For this review, take the finished solid that the model builds, in its own axes (mm). A direction names the side the tool comes from. Give positions to 0.01 mm unless a question says otherwise; leave off trailing zeros. Loops run counter-clockwise (first coordinate to the right, second up) from the corner with the lowest first, then second, coordinate; pieces in that order, holes last.
Autodesk Inventor part; units mm, degrees
ref_plane "YZ Plane" through (0, 0, 0) normal (1, 0, 0) x (0, 1, 0)
ref_plane "XZ Plane" through (0, 0, 0) normal (0, 1, 0) x (-1, 0, 0)
ref_plane "XY Plane" through (0, 0, 0) normal (0, 0, 1) x (1, 0, 0)
sketch "Sketch1" plane through (0, 0, 0) normal (1, 0, 0) x (0, 1, 0)
  line L0 (0, 0) -> (40, 0) construction
  line L1 (40, 0) -> (40, 66.5) construction
  line L2 (40, 66.5) -> (0, 66.5) construction
  line L3 (0, 66.5) -> (0, 0) construction
  line L4 (0, 66.5) -> (40, 66.5) construction
  line L5 (40, 66.5) -> (40, 86.5) construction
  line L6 (40, 86.5) -> (0, 86.5)
  line L7 (0, 86.5) -> (0, 66.5) construction
  line L8 (0, 0) -> (40, 0) construction
  line L9 (40, 0) -> (40, -20) construction
  line L10 (40, -20) -> (0, -20) construction
  line L11 (0, -20) -> (0, 0) construction
  line L12 (48.2, 61.45) -> (-8.2, 61.45) construction
  line L13 (-8.2, 61.45) -> (-8.2, 5.05) construction
  line L14 (-8.2, 5.05) -> (48.2, 5.05) construction
  line L15 (48.2, 5.05) -> (48.2, 61.45) construction
  line L16 (48.2, 33.25) -> (-8.2, 33.25) construction
  line L17 (40, 33.25) -> (0, 33.25) construction
  line L18 (43.57, 56.82) -> (-3.57, 56.82) construction
  line L19 (-3.57, 56.82) -> (-3.57, 9.68) construction
  line L20 (-3.57, 9.68) -> (43.57, 9.68) construction
  line L21 (43.57, 9.68) -> (43.57, 56.82) construction
  line L22 (43.57, 56.82) -> (48.2, 56.82) construction
  line L23 (43.57, 56.82) -> (43.57, 61.45) construction
  line L24 (-3.57, 9.68) -> (-8.2, 9.68) construction
  line L25 (-3.57, 9.68) -> (-3.57, 5.05) construction
  line L26 (40, -10) -> (0, -10) construction
  line L27 (40, 76.5) -> (0, 76.5) construction
  circle A0 centre (30, 76.5) radius 2.1
  circle A1 centre (10, 76.5) radius 2.1
  circle A2 centre (30, -10) radius 2.1
  circle A3 centre (10, -10) radius 2.1
  circle A4 centre (43.57, 56.82) radius 2.6
  circle A5 centre (43.57, 9.68) radius 2.6
  circle A6 centre (-3.57, 9.68) radius 2.6
  circle A7 centre (-3.57, 56.82) radius 2.6
  circle A8 centre (20, 33.25) radius 19.15
  circle A9 centre (-25, 18.25) radius 11.08 construction
  circle A10 centre (-25, 18.25) radius 13 construction
  circle A11 centre (-25, 18.25) radius 2.5
  line L28 (-60, 153.25) -> (-60, -86.75) construction
  circle A12 centre (-60, -86.75) radius 2.6
  circle A13 centre (-60, 153.25) radius 2.6
  line L29 (-120.2, 153.25) -> (-120.2, -86.75) construction
  circle A14 centre (-120.2, -86.75) radius 2.6
  circle A15 centre (-120.2, 153.25) radius 2.6
  circle A16 centre (-60, -86.75) radius 12 construction
  circle A17 centre (-120.2, -86.75) radius 12 construction
  circle A18 centre (-120.2, 153.25) radius 12 construction
  circle A19 centre (-60, 153.25) radius 12 construction
  line L30 (-110, 482.7599) -> (-70, 482.7599) construction
  line L31 (-70, -517.2401) -> (-110, -517.2401) construction
  circle A20 centre (-25, 48.25) radius 2.5
  circle A21 centre (-25, 48.25) radius 11.08 construction
  circle A22 centre (-25, 48.25) radius 13 construction
  circle A23 centre (20, 33.25) radius 11.08 construction
  circle A24 centre (20, 33.25) radius 13 construction
  line L32 (-23.1873, 29.1807) -> (18.1873, 22.3193) construction
  line L33 (18.1873, 44.1807) -> (-23.1873, 37.3193) construction
  line L34 (-120.8333, -99.25) -> (-47.8333, -99.25)
  line L35 (-47.8333, 165.75) -> (-120.8333, 165.75)
  line L36 (-132.8333, 153.75) -> (-132.8333, -87.25)
  line L37 (-60, 153.25) -> (-120.2, 153.25) construction
  line L38 (-120.2, -86.75) -> (-60, -86.75) construction
  line L39 (-60, 153.25) -> (-60, 165.75) construction
  line L40 (-120.2, -86.75) -> (-120.2, -99.25) construction
  line L41 (48.3276, -20) -> (48.3276, 86.5)
  line L42 (17.6122, 86.5) -> (40, 86.5) construction
  arc A25 (-120.8333, 165.75) -> (-132.8333, 153.75) centre (-120.8333, 153.75) ccw
  arc A26 (-132.8333, -87.25) -> (-120.8333, -99.25) centre (-120.8333, -87.25) ccw
  line L43 (48.3276, -20) -> (-47.8333, -99.25)
  line L44 (-47.8333, 165.75) -> (-47.8333, -99.25) construction
  line L45 (-120.2, -86.75) -> (-132.8333, -86.75) construction
  line L46 (-60, 153.25) -> (-47.8333, 153.25) construction
  line L47 (-36.08, 48.25) -> (-36.08, 286.613) construction
  line L48 (-47.8333, 145.75) -> (-47.8333, 86.5)
  line L49 (-47.8333, 86.5) -> (16.8804, 86.5)
  line L50 (-47.8333, -73.3332) -> (16.8804, -20)
  line L51 (-47.8333, -73.3332) -> (-47.8333, -20)
  line L52 (-47.8333, -20) -> (16.8804, -20)
  line L53 (48.3276, 86.5) -> (48.3276, 165.75)
  line L54 (48.3276, 165.75) -> (-47.8333, 165.75)
  line L55 (-47.8333, 145.75) -> (28.3276, 145.75)
  line L56 (28.3276, 145.75) -> (28.3276, 86.5)
  line L57 (-47.8333, 145.75) -> (28.3276, 86.5) construction
  line L58 (-39.6904, 145.75) -> (28.3276, 92.8349)
  line L59 (-47.8333, 139.4151) -> (20.1847, 86.5)
  point P0 (-132.8333, -99.25)
  point P1 (-132.8333, 165.75)
  point P2 (-47.8333, 139.8332)
  point P3 (0, 86.5)
  dimension "d25" = 22.16
  dimension "d0" = 40
  dimension "d1" = 66.5
  dimension "d2" = 40
  dimension "d3" = 20
  dimension "d4" = 40
  dimension "d5" = 20
  dimension "d6" = 56.4
  dimension "d7" = 56.4
  dimension "d8" = 0
  dimension "d9" = 8.2
  dimension "d10" = 47.14
  dimension "d11" = 47.14
  dimension "d12" = 4.2
  dimension "d13" = 20
  dimension "d14" = 10
  dimension "d15" = 10
  dimension "d16" = 20
  dimension "d17" = 4.2
  dimension "d18" = 4.2
  dimension "d19" = 4.2
  dimension "d20" = 5.2
  dimension "d21" = 5.2
  dimension "d22" = 5.2
  dimension "d23" = 5.2
  dimension "d24" = 38.3
  dimension "d26" = 26
  dimension "d27" = 5
  dimension "d28" = 240
  dimension "d30" = 60
  dimension "d31" = 5.2
  dimension "d32" = 5.2
  dimension "d33" = 5.2
  dimension "d34" = 5.2
  dimension "d35" = 60.2
  dimension "d36" = 24
  dimension "d37" = 24
  dimension "d38" = 24
  dimension "d39" = 24
  dimension "d40" = 40
  dimension "d41" = 1000
  dimension "d44" = 45
  dimension "d45" = 5
  dimension "d46" = 22.16
  dimension "d47" = 26
  dimension "d48" = 45
  dimension "d49" = 22.16
  dimension "d50" = 26
  dimension "d51" = 15
  dimension "d52" = 15
  dimension "d53" = 265
  dimension "d54" = 85
  dimension "d55" = 106.5
  dimension "d60" = 12
  dimension "d84" = 72.8333
  dimension "d87" = 28.3276
  dimension "d90" = 53.25
  dimension "d91" = 85
  dimension "d92" = 132.5
  dimension "d93" = 60.2
  dimension "d99" = 20
  dimension "d100" = 20
  dimension "d102" = 5
  dimension "d103" = 5
extrude "Extrusion1" add sketch "Sketch1" along normal blind 3.175 contours L6 L59 L48 L55 L58 L56 | A26 L36 A25 L35 L54 L53 L41 L43 L34
sketch "Sketch4" plane through (3.175, 0, 0) normal (1, 0, 0) x (0, 0, -1)
  line L0 (20, 16.8804) -> (73.3332, -47.8333)
  line L1 (20, 16.8804) -> (73.3332, -47.8333)
  line L2 (39.0796, -6.2705) -> (54.5136, 6.4492) construction
  line L3 (99.25, -47.8333) -> (20, 48.3276)
  circle A0 centre (37.2568, 11.6648) radius 2.6
  circle A1 centre (56.3364, -11.4861) radius 2.6
  line L4 (37.2568, 11.6648) -> (46.7966, 0.0893) construction
  line L5 (56.3364, -11.4861) -> (46.7966, 0.0893) construction
  line L6 (-145.75, 28.3276) -> (-92.8349, 28.3276)
  line L7 (-119.2924, 28.3276) -> (-119.2924, 48.3276) construction
  line L8 (20, 48.3276) -> (-165.75, 48.3276) construction
  circle A2 centre (-104.2924, 38.3276) radius 2.6
  circle A3 centre (-134.2924, 38.3276) radius 2.6
  line L9 (-104.2924, 38.3276) -> (-119.2924, 38.3276) construction
  line L10 (-134.2924, 38.3276) -> (-119.2924, 38.3276) construction
  point P0 (0, 0)
  dimension "d107" = 5.2
  dimension "d108" = 5.2
  dimension "d109" = 15
  dimension "d110" = 15
  dimension "d111" = 30
  dimension "d112" = 5.2
  dimension "d113" = 5.2
  dimension "d114" = 15
  dimension "d115" = 15
extrude "Extrusion4" cut sketch "Sketch4" against normal through all
fillet "Fillet2" radius 3.175 7 edges at (1.5875, -47.8333, 139.4151) (1.5875, -47.8333, 86.5) (1.5875, -47.8333, -20) (1.5875, -47.8333, -73.3332) (1.5875, 16.8804, -20) (1.5875, 48.3276, -20) (1.5875, -47.8333, -99.25)
fillet "Fillet3" radius 3.175 4 edges at (1.5875, 28.3276, 145.75) (1.5875, 28.3276, 92.8349) (1.5875, 20.1847, 86.5) (1.5875, -39.6904, 145.75)
chamfer "Chamfer1" distance 10 angle 45 1 edges at (1.5875, 48.3276, 165.75)
equation "\"d11\" = d10"
equation "\"d17\" = d12"
equation "\"d18\" = d12"
equation "\"d19\" = d12"
equation "\"d21\" = d20"
equation "\"d22\" = d20"
equation "\"d23\" = d20"
equation "\"d32\" = d31"
equation "\"d33\" = d31"
equation "\"d34\" = d31"
equation "\"d37\" = d36"
equation "\"d38\" = d36"
equation "\"d39\" = d36"
equation "\"d45\" = d27"
equation "\"d46\" = d25"
equation "\"d47\" = d26"
properties part number "X Axis V Wheel and Motor Frame Machined"
Item 1: Take a section at B-B on z = 123.5. Give the boundary of the cut face in (x, y) (3 decimals).
Answer:
outline: (0, -132.833) - (3.175, -132.833) - (3.175, -47.833) - (0, -47.833) - close; (0, -27.376) - (3.175, -27.376) - (3.175, -11.09) - (0, -11.09) - close; (0, 28.328) - (3.175, 28.328) - (3.175, 48.328) - (0, 48.328) - close
Item 2: Tool access review of faces 1 (the flat face through (1.565, -15.302, 114.107)), 2 (the flat face through (0, -64, 35)): name each direction out of +Z, -Z, +X, -X, +Y, -Y from which nothing blocks a thin tool from reaching the whole face with its end or side.
Answer:
face 1: +X, -X
face 2: +Z, -Z, -X, +Y, -Y
Item 3: The part is to be moulded in two halves that separate along Y. For faces 3 (the cylindrical face through (1.565, -129.411, 162.141)), 4 (the flat face through (3.175, -64, 35)), 5 (the cylindrical face through (1.6, -3.9, 7.1)), say which applies: released by +Y, released by -Y, zero draft, split by the parting line, or undercut.
Answer:
face 3: released by -Y
face 4: zero draft
face 5: undercut
Item 4: Take a section at D-D on z = -46. Give the boundary of the cut face in (x, y) (3 decimals).
Answer:
outline: (0, -132.833) - (3.175, -132.833) - (3.175, -47.833) - (0, -47.833) - close; (0, -14.668) - (3.175, -14.668) - (3.175, 16.78) - (0, 16.78) - close
Item 5: Take a section at C-C on y = -3.57. Give the boundary of the cut face in (x, z) (3 decimals).
Answer:
outline: (0, -62.771) - (3.175, -62.771) - (3.175, -36.854) - (0, -36.854) - close; (0, -20) - (3.175, -20) - (3.175, 7.08) - (0, 7.08) - close; (0, 12.28) - (3.175, 12.28) - (3.175, 54.22) - (0, 54.22) - close; (0, 59.42) - (3.175, 59.42) - (3.175, 86.5) - (0, 86.5) - close; (0, 104.98) - (3.175, 104.98) - (3.175, 117.65) - (0, 117.65) - close; (0, 145.75) - (3.175, 145.75) - (3.175, 165.75) - (0, 165.75) - close
Item 6: For L1, parallel to Z at x = 2.1, y = 13.5; L2, parallel to Z at x = 1.2, y = 20; L3, parallel to Y at x = 2.25, z = 134.5, list the stretches that pass through material, from the lowest coordinate up.
Answer:
L1: z = -48.7 to -39.1, -35.42 to 15.24, 51.26 to 87.81, 91.54 to 104.37, 145.75 to 165.75
L2: z = -43.35 to 14.1, 52.4 to 99.31, 145.75 to 165.75
L3: y = -132.83 to -47.41, -41.52 to -25.23, 28.33 to 35.74, 40.92 to 48.33
Item 7: Clearance check with flat-ended pins moving along their axes: pin 1 Ø4 at (y, z) = (-25, 18.25) entering from -X; pin 2 Ø1.6 at (x, y) = (1.5, -31) entering from -Z; pin 3 Ø1 at (x, z) = (2.5, -44) entering from +Y; pin 4 Ø8.5 at (y, z) = (-11.49, -56.34) entering from -X. State where each tip first meets the part, or that it passes through.
Answer:
pin 1: passes through
pin 2: stops at z = -86.04
pin 3: stops at y = 19.81
pin 4: stops at x = 0
Item 8: Take a section at A-A on y = 20. Give the boundary of the cut face in (x, z) (3 decimals), and give its area (3 significant figures).
Answer:
outline: (0, -43.346) - (3.175, -43.346) - (3.175, 14.1) - (0, 14.1) - close; (0, 52.4) - (3.175, 52.4) - (3.175, 99.313) - (0, 99.313) - close; (0, 145.75) - (3.175, 145.75) - (3.175, 165.75) - (0, 165.75) - close
area: 395 mm2
